```python
from build123d import *
from build123d.topology import SkipClean

# Parameters (mm, degrees)
SKETCH_1_R                   = 26.5
EXTRUDE_1_DEPTH              = 5
HOLE_WIZARD_M4_1_AT_2_COUNT  = 2
HOLE_WIZARD_M4_1_AT_2_PITCH  = 39.424388736
HOLE_WIZARD_M4_1_AT_3_COUNT  = 2
HOLE_WIZARD_M4_1_AT_3_PITCH  = 39.424388736
HOLE_WIZARD_M4_1_AT_4_COUNT  = 2
HOLE_WIZARD_M4_1_AT_4_PITCH  = 18.383894388
HOLE_WIZARD_M4_1_AT_5_COUNT  = 2
HOLE_WIZARD_M4_1_AT_5_PITCH  = 43.5
HOLE_WIZARD_M4_1_AT_6_COUNT  = 2
HOLE_WIZARD_M4_1_AT_6_PITCH  = 39.424388736
HOLE_WIZARD_M4_1_AT_7_COUNT  = 2
HOLE_WIZARD_M4_1_AT_7_PITCH  = 18.383894388
EXTRUDE_1551_DEPTH           = 8
CUT_EXTRUDE_START            = 22
SKETCH_6_R                   = 4
CUT_EXTRUDE_1661_DEPTH       = 22
SKETCH_8_R                   = 34.5
CUT_EXTRUDE_1747_DEPTH       = 119.962346984
HOLE_WIZARD_M3_1_D           = 3.4
HOLE_WIZARD_M3_1_CBORE_D     = 6.5
HOLE_WIZARD_M3_1_CBORE_DEPTH = 3
CUT_EXTRUDE_1_DEPTH          = 15
CUT_EXTRUDE_2_DEPTH          = 5
CUT_EXTRUDE_3_DEPTH          = 10
SKETCH_15_W                  = 96
SKETCH_15_H                  = 8
CUT_EXTRUDE_4_DEPTH          = 113.29536945
CUT_EXTRUDE_5_DEPTH          = 10


with BuildPart() as part:
    # Sketch 1 → Extrude 1 (new body)
    with BuildSketch(Plane.XY):
        Circle(SKETCH_1_R)
    extrude(amount=EXTRUDE_1_DEPTH)

    # Sketch 3 → Hole Wizard M4 _1 (revolve, cut)
    with BuildSketch(Plane(origin=(21.75, 0, 5), x_dir=(0, -1, 0), z_dir=(1, 0, 0))):
        Polygon((0, 0), (0, 5), (2.25, 5), (2.25, 4), (4, 4), (4, 0), align=None)
    hole_wizard_m4_1 = revolve(axis=Axis((21.75, 0, 11.35), (0, 0, -1)), mode=Mode.SUBTRACT)

    # Hole Wizard M4 _1 at 2: Hole Wizard M4 _1 ×2
    with Locations(*[Vector(-0.9063077870366496, 0.4226182617407002, 0) * (i * HOLE_WIZARD_M4_1_AT_2_PITCH) for i in range(1, HOLE_WIZARD_M4_1_AT_2_COUNT)]):
        add(hole_wizard_m4_1, mode=Mode.SUBTRACT)

    # Hole Wizard M4 _1 at 3: Hole Wizard M4 _1 ×2
    with Locations(*[Vector(-0.9063077870125524, 0.42261826179237694, 0) * (i * HOLE_WIZARD_M4_1_AT_3_PITCH) for i in range(1, HOLE_WIZARD_M4_1_AT_3_COUNT)]):
        add(hole_wizard_m4_1, mode=Mode.SUBTRACT)

    # Hole Wizard M4 _1 at 4: Hole Wizard M4 _1 ×2
    with Locations(*[Vector(-0.42261826172613215, 0.9063077870434428, 0) * (i * HOLE_WIZARD_M4_1_AT_4_PITCH) for i in range(1, HOLE_WIZARD_M4_1_AT_4_COUNT)]):
        add(hole_wizard_m4_1, mode=Mode.SUBTRACT)

    # Hole Wizard M4 _1 at 5: Hole Wizard M4 _1 ×2
    with Locations(*[(-i * HOLE_WIZARD_M4_1_AT_5_PITCH, 0, 0) for i in range(1, HOLE_WIZARD_M4_1_AT_5_COUNT)]):
        add(hole_wizard_m4_1, mode=Mode.SUBTRACT)

    # Hole Wizard M4 _1 at 6: Hole Wizard M4 _1 ×2
    with Locations(*[Vector(-0.9063077870125524, -0.42261826179237694, 0) * (i * HOLE_WIZARD_M4_1_AT_6_PITCH) for i in range(1, HOLE_WIZARD_M4_1_AT_6_COUNT)]):
        add(hole_wizard_m4_1, mode=Mode.SUBTRACT)

    # Hole Wizard M4 _1 at 7: Hole Wizard M4 _1 ×2
    with Locations(*[Vector(-0.42261826172613215, -0.9063077870434428, 0) * (i * HOLE_WIZARD_M4_1_AT_7_PITCH) for i in range(1, HOLE_WIZARD_M4_1_AT_7_COUNT)]):
        add(hole_wizard_m4_1, mode=Mode.SUBTRACT)

    # Sketch 5 → Extrude 1551 (add)
    with BuildSketch(Plane.XZ.offset(-8.7)):
        with BuildLine():
            Line((-26.5, 5), (-26.5, 14.978130978))
            ThreePointArc((-26.5, 14.978130978), (0, 103), (26.5, 14.978130978))
            Line((26.5, 14.978130978), (26.5, 5))
            Line((26.5, 5), (-26.5, 5))
        make_face()
    extrude(amount=-EXTRUDE_1551_DEPTH)

    # Sketch 6 → Cut-Extrude 1661 (cut)
    with SkipClean():  # the faces are left unmerged after this step: merging them gives an invalid solid
        with BuildSketch(Plane.XY.offset(5).offset(CUT_EXTRUDE_START)):
            with Locations((-13.98063051, 16.66146664)):
                Circle(SKETCH_6_R)
            with Locations((13.98063051, 16.66146664)):
                Circle(SKETCH_6_R)
        extrude(amount=-CUT_EXTRUDE_1661_DEPTH, mode=Mode.SUBTRACT)
    add(part.part.scale(1), mode=Mode.REPLACE)  # the faces are merged on a copy

    # Sketch 8 → Cut-Extrude 1747 (cut, through all)
    with BuildSketch(Plane.XZ.offset(-8.7)):
        with Locations(Location((0, 55, 0), (0, 0, 270))):
            Circle(SKETCH_8_R)
    extrude(amount=-CUT_EXTRUDE_1747_DEPTH, mode=Mode.SUBTRACT)

    # Hole Wizard M3 _1 (through all)
    with Locations(Plane(origin=(-9.576304669, 16.7, 19.260744427), x_dir=(0, 0, 1), z_dir=(0, 1, 0))):
        with Locations((0, 0), (0, 19.152609338), (9.576304669, 35.739255573), (26.162950904, 45.315560242), (45.315560242, 45.315560242), (62.358629164, 36.19567826), (71.478511143, 19.152609339), (71.478511146, 0), (61.902206477, -16.586646235), (9.576304669, -16.586646235), (26.162950904, -26.162950904), (45.315560242, -26.162950904)):
            CounterBoreHole(HOLE_WIZARD_M3_1_D / 2, HOLE_WIZARD_M3_1_CBORE_D / 2, HOLE_WIZARD_M3_1_CBORE_DEPTH)

    # Sketch 11 → Cut-Extrude 1 (cut)
    with BuildSketch(Plane.XY):
        with BuildLine():
            Line((-25.031180555, 8.7), (-29.031180555, 8.7))
            Line((-29.031180555, 8.7), (-29.031180555, 16.7))
            Line((-29.031180555, 16.7), (-20.575713839, 16.7))
            ThreePointArc((-20.575713839, 16.7), (-23.151613423, 12.893905379), (-25.031180555, 8.7))
        make_face()
        with BuildLine():
            Line((29.031180555, 16.7), (20.575713839, 16.7))
            ThreePointArc((20.575713839, 16.7), (23.151613423, 12.893905379), (25.031180555, 8.7))
            Line((25.031180555, 8.7), (29.031180555, 8.7))
            Line((29.031180555, 8.7), (29.031180555, 16.7))
        make_face()
    extrude(amount=CUT_EXTRUDE_1_DEPTH, mode=Mode.SUBTRACT)

    # Sketch 12 → Cut-Extrude 2 (cut)
    with BuildSketch(Plane.XZ.offset(-8.7)):
        with BuildLine():
            Line((30.640436297, 73.992699353), (39.299497484, 79.033088453))
            ThreePointArc((39.299497484, 79.033088453), (22.961941343, 94.93481054), (1, 101.054748323))
            Line((1, 101.054748323), (1, 96.032801673))
            Line((1, 96.032801673), (1, 90.986108088))
            ThreePointArc((1, 90.986108088), (3.29678588, 90.848726312), (5.580104544, 90.56490417))
            ThreePointArc((5.580104544, 90.56490417), (10.611585442, 94.602959438), (12.949935188, 88.59015553))
            ThreePointArc((12.949935188, 88.59015553), (18.110429302, 86.112886725), (22.813026139, 82.848971404))
            ThreePointArc((22.813026139, 82.848971404), (29.429042421, 84.466469087), (27.899229179, 77.829629354))
            ThreePointArc((27.899229179, 77.829629354), (29.332637394, 75.956033707), (30.640436297, 73.992699353))
        make_face()
        with BuildLine():
            Line((40.299497484, 32.887774818), (31.628764833, 37.893824648))
            ThreePointArc((31.628764833, 37.893824648), (32.656681203, 39.948715244), (33.551263667, 42.065058704))
            ThreePointArc((33.551263667, 42.065058704), (39.60579141, 44.366506044), (35.564535509, 49.428345312))
            ThreePointArc((35.564535509, 49.428345312), (35.998326415, 55.004146142), (35.563251124, 60.5798469))
            ThreePointArc((35.563251124, 60.5798469), (39.603491283, 65.610874453), (33.58998558, 67.95021794))
            ThreePointArc((33.58998558, 67.95021794), (32.667369713, 70.12740004), (31.60381627, 72.239317654))
            Line((31.60381627, 72.239317654), (40.220731453, 77.255173811))
            ThreePointArc((40.220731453, 77.255173811), (45.9673073, 55.081606369), (40.299497484, 32.887774818))
        make_face()
        with BuildLine():
            Line((25.409425198, 16.693850218), (19.898823765, 25.001394455))
            ThreePointArc((19.898823765, 25.001394455), (21.276296399, 25.962115548), (22.607462255, 26.98603612))
            ThreePointArc((22.607462255, 26.98603612), (29.011771602, 26.01712548), (27.977619592, 32.411223983))
            ThreePointArc((27.977619592, 32.411223983), (29.36313556, 34.244126853), (30.628764833, 36.161773841))
            Line((30.628764833, 36.161773841), (39.299497484, 31.15572401))
            ThreePointArc((39.299497484, 31.15572401), (33.152641178, 23.15816615), (25.409425198, 16.693850218))
        make_face()
        with BuildLine():
            Line((-1, 90.986108088), (-1, 96.032801673))
            Line((-1, 96.032801673), (-1, 101.054748323))
            ThreePointArc((-1, 101.054748323), (-22.961941343, 94.93481054), (-39.299497484, 79.033088453))
            Line((-39.299497484, 79.033088453), (-30.640436297, 73.992699353))
            ThreePointArc((-30.640436297, 73.992699353), (-29.332637394, 75.956033707), (-27.899229179, 77.829629354))
            ThreePointArc((-27.899229179, 77.829629354), (-29.429042421, 84.466469087), (-22.813026139, 82.848971404))
            ThreePointArc((-22.813026139, 82.848971404), (-18.110429302, 86.112886725), (-12.949935188, 88.59015553))
            ThreePointArc((-12.949935188, 88.59015553), (-10.611585442, 94.602959438), (-5.580104544, 90.56490417))
            ThreePointArc((-5.580104544, 90.56490417), (-3.29678588, 90.848726312), (-1, 90.986108088))
        make_face()
        with BuildLine():
            ThreePointArc((-31.628764833, 37.893824648), (-32.656681203, 39.948715244), (-33.551263667, 42.065058704))
            ThreePointArc((-33.551263667, 42.065058704), (-39.60579141, 44.366506044), (-35.564535509, 49.428345312))
            ThreePointArc((-35.564535509, 49.428345312), (-35.998326415, 55.004146142), (-35.563251124, 60.5798469))
            ThreePointArc((-35.563251124, 60.5798469), (-39.603491283, 65.610874453), (-33.58998558, 67.95021794))
            ThreePointArc((-33.58998558, 67.95021794), (-32.667369713, 70.12740004), (-31.60381627, 72.239317654))
            Line((-31.60381627, 72.239317654), (-40.220731453, 77.255173811))
            ThreePointArc((-40.220731453, 77.255173811), (-45.9673073, 55.081606369), (-40.299497484, 32.887774818))
            Line((-40.299497484, 32.887774818), (-31.628764833, 37.893824648))
        make_face()
        with BuildLine():
            ThreePointArc((-22.607462255, 26.98603612), (-21.276296399, 25.962115548), (-19.898823765, 25.001394455))
            Line((-19.898823765, 25.001394455), (-25.409425198, 16.693850218))
            ThreePointArc((-25.409425198, 16.693850218), (-33.152641178, 23.15816615), (-39.299497484, 31.15572401))
            Line((-39.299497484, 31.15572401), (-30.628764833, 36.161773841))
            ThreePointArc((-30.628764833, 36.161773841), (-29.36313556, 34.244126853), (-27.977619592, 32.411223983))
            ThreePointArc((-27.977619592, 32.411223983), (-29.011771602, 26.01712548), (-22.607462255, 26.98603612))
        make_face()
    extrude(amount=-CUT_EXTRUDE_2_DEPTH, mode=Mode.SUBTRACT)

    # Sketch 13 → Cut-Extrude 3 (cut)
    with BuildSketch(Plane.XY.offset(5)):
        with BuildLine():
            Line((-12.219247113, 8.7), (12.219247113, 8.7))
            ThreePointArc((12.219247113, 8.7), (0, -15), (-12.219247113, 8.7))
        make_face()
    extrude(amount=-CUT_EXTRUDE_3_DEPTH, mode=Mode.SUBTRACT)

    # Sketch 15 → Cut-Extrude 4 (cut, through all)
    with BuildSketch(Plane.XY.offset(5)):
        with Locations((0, 12.7)):
            Rectangle(SKETCH_15_W, SKETCH_15_H)
    extrude(amount=CUT_EXTRUDE_4_DEPTH, mode=Mode.SUBTRACT)

    # Sketch 17 → Cut-Extrude 5 (cut)
    with BuildSketch(Plane.XY.offset(5)):
        Polygon((0, 12.7), (-9, 12.7), (-9, 16.7), (9, 16.7), (9, 12.7), align=None)
    extrude(amount=-CUT_EXTRUDE_5_DEPTH, mode=Mode.SUBTRACT)


solid = part.part
```
The model under review builds one solid part; all positions refer to its coordinate system, in mm. A direction names the side the tool comes from. Give positions to 0.01 mm unless a question says otherwise; leave off trailing zeros. Write each loop counter-clockwise with the first axis right and the second up, starting at its lowest first coordinate (ties: lowest second). Pieces come first, ordered by that corner, then holes. Notation, with made-up numbers: M 69,24 L 109,24 A27 ccw 109,61 Z; hole C -33,-32.75 d6. An arc over 180 degrees is marked long. Answer in a Markdown table with one row per item.
Item 1: Add section A-A on y = 0. Give the boundary of the cut face in (x, z), plus the area to 3 significant figures.
Check sheet entries:
| item | result |
|---|---|
| outline | M -26.5,0 L -24,0 L -24,1 L -25.75,1 L -25.75,5 L -26.5,5 Z; M -19.5,0 L -15,0 L -15,5 L -17.75,5 L -17.75,1 L -19.5,1 Z; M 15,0 L 19.5,0 L 19.5,1 L 17.75,1 L 17.75,5 L 15,5 Z; M 24,0 L 26.5,0 L 26.5,5 L 25.75,5 L 25.75,1 L 24,1 Z |
| area | 42.0 mm2 |
Item 2: Add section B-B on x = 0. Give the boundary of the cut face in (y, z), plus the area to 4 significant figures.
Check sheet entries:
| item | result |
|---|---|
| outline | M -26.5,0 L -15,0 L -15,5 L -26.5,5 Z; M 8.7,0 L 12.7,0 L 12.7,5 L 8.7,5 Z; M 16.7,0 L 26.5,0 L 26.5,5 L 16.7,5 Z |
| area | 126.5 mm2 |
Item 3: For P1, Ø7, axis at x = 13.98, y = -16.66, coming from the +Z side; P2, Ø1.5, axis at y = -11, z = 1.5, coming from the -X side; P3, Ø2.5, axis at x = -14, y = -16, coming from the +Z side; P4, Ø3, axis at y = -6, z = 1, coming from the +X side, all flat-tipped, find the tip position at first contact; note any pin that passes through.
Check sheet entries:
| item | result |
|---|---|
| P1 | z = 1 |
| P2 | x = -24.44 |
| P3 | through |
| P4 | x = 26.12 |
Item 4: Tool access review of faces 4 (the face through (23.5, 1.7, 1)), 5 (the face through (0, 8.7, 3)), 6 (the face through (0, 12, 0)): name each direction out of +Z, -Z, +X, -X, +Y, -Y from which nothing blocks a thin tool from reaching the whole face with its end or side.
Check sheet entries:
| item | result |
|---|---|
| face 4 | +Z |
| face 5 | +Z, -Z |
| face 6 | -Z, +X, -X, +Y, -Y |
Item 5: Add section C-C on y = -12. Give the boundary of the cut face in (x, z).
Check sheet entries:
| item | result |
|---|---|
| outline | M -23.63,0 L -9,0 L -9,5 L -23.63,5 Z; M 9,0 L 23.63,0 L 23.63,5 L 9,5 Z |
Item 6: For line 1 along Y through (x, z) = (0, 3.35); line 2 along Y through (x, z) = (3.5, 3.35); line 3 along X through (y, z) = (-17, 1.15), list the stretches that pass through material, from the lowest coordinate up.
Check sheet entries:
| item | result |
|---|---|
| line 1 | -26.5 to -15, 8.7 to 12.7, 16.7 to 26.5 |
| line 2 | -26.27 to -14.59, 8.7 to 12.7, 16.7 to 26.27 |
| line 3 | -20.33 to -17.97, -9.99 to 9.99, 17.97 to 20.33 |
Item 7: Add section D-D on x = -21.75. Give the boundary of the cut face in (y, z), plus the area to 3 significant figures.
Check sheet entries:
| item | result |
|---|---|
| outline | M -15.14,0 L -2.25,0 L -2.25,1 L -4,1 L -4,5 L -15.14,5 Z; M 2.25,0 L 15.14,0 L 15.14,5 L 4,5 L 4,1 L 2.25,1 Z |
| area | 115 mm2 |
Item 8: Draft analysis for pull direction Y (two halves, no side actions). For faces 1 (the face through (0, 16.7, 3)), 2 (the face through (14.246, 22.345, 2.465)), 3 (the face through (0, 12, 5)), state which applies: +Y half, -Y half, draft (parallel to the pull), parting line (faces both ways), or undercut.
Check sheet entries:
| item | result |
|---|---|
| face 1 | undercut |
| face 2 | parting line |
| face 3 | draft |
